from build123d import *

# Parameters (mm, degrees)
F0_W        = 292.1
F0_H        = 474.98
F1_DEPTH    = 12.7
F2_W        = 157.1649909019
F2_H        = 403.2308459282
F3_DEPTH    = 6.35
F4_T1_DEPTH = 445.8279408996
F4_T3_DEPTH = 199.7620858733


# Not quite as in the source:
# - a fillet or chamfer that OpenCascade refuses, or shapes differently, is made with other operations: its cross-section is extruded or revolved along the edge and cut away or added


with BuildPart() as f1:
    # F0 (on Front) → F1 (new body)
    with BuildSketch(Plane.XZ):
        Rectangle(F0_W, F0_H)
    extrude(amount=F1_DEPTH)

    # F2 (on face) → F3 (cut)
    with BuildSketch(Plane.XZ.offset(12.7)):
        Rectangle(F2_W, F2_H)
    extrude(amount=-F3_DEPTH, mode=Mode.SUBTRACT)

    # F4: fillet of radius 8.89 on 4 edges, made by hand

    # F4_s2 → F4_t1 (join)
    with BuildSketch(Plane.XY.offset(-222.9139704498)):
        with BuildLine():
            ThreePointArc((78.582495451, -12.7), (75.3758676252, -8.1121426782), (70.0630764567, -6.35))
            Line((70.0630764567, -6.35), (78.582495451, -6.35))
            Line((78.582495451, -6.35), (78.582495451, -12.7))
        make_face()
        with BuildLine():
            ThreePointArc((-78.582495451, -12.7), (-75.3758676252, -8.1121426782), (-70.0630764567, -6.35))
            Line((-70.0630764567, -6.35), (-78.582495451, -6.35))
            Line((-78.582495451, -6.35), (-78.582495451, -12.7))
        make_face()
    extrude(amount=F4_T1_DEPTH)

    # F4_s4 → F4_t3 (join)
    with BuildSketch(Plane.YZ.offset(-99.8810429367)):
        with BuildLine():
            ThreePointArc((-12.7, 201.6154229641), (-8.1121426782, 198.4087951383), (-6.35, 193.0960039698))
            Line((-6.35, 193.0960039698), (-6.35, 201.6154229641))
            Line((-6.35, 201.6154229641), (-12.7, 201.6154229641))
        make_face()
        with BuildLine():
            ThreePointArc((-12.7, -201.6154229641), (-8.1121426782, -198.4087951383), (-6.35, -193.0960039698))
            Line((-6.35, -193.0960039698), (-6.35, -201.6154229641))
            Line((-6.35, -201.6154229641), (-12.7, -201.6154229641))
        make_face()
    extrude(amount=F4_T3_DEPTH)


solid = f1.part
Model file for the job. Use its own axes, mm. A direction names the side the tool comes from. Coordinates: 2 decimals unless noted, no trailing zeros. Write each loop counter-clockwise with the first axis right and the second up, starting at its lowest first coordinate (ties: lowest second). Pieces come first, ordered by that corner, then holes. Notation, with made-up numbers: (78.5, 40.25) -> (113.5, 40.25) arc R26 cw to (113.5, 68.25) -> close; hole circle Ø4 at (-11, 38.25). An arc over 180 degrees is marked (long way). One line per item, written item: value. Start each with the question number.
1) Which spindle directions (+Z, -Z, +X, -X, +Y, -Y) get a long thin tool onto all of the face, cutting with end or side? Do faces 1 (the face through (-2, 0, 3)), 2 (the face through (-1.1, -8.16, 198.47)). Say none if no direction does.
2) Slice it at B-B on z = -110.5. Write the cut outline in (x, y), then the cut area to 3 significant figures.
3) Probe probe 1 along Y at (x, z) = (-39, 30); probe 2 along X at (y, z) = (-7.25, 107); probe 3 along X at (y, z) = (-8, 124). List the from-to ranges inside material, lowest first.
4) Flat gauge pins, fed straight in: pin 1 Ø6 at (x, z) = (28.5, 188) entering from -Y; pin 2 Ø1.5 at (x, z) = (-76, 89.5) entering from -Y. Where does each tip first touch, or does it go through?
5) Slice it at C-C on y = -9. Write the cut outline in (x, z), then the cut area to 3 significant figures.
6) Slice it at A-A on x = -53.5. Write the cut outline in (y, z), then the cut area to 3 significant figures.
7) Pull direction Z, two halves, no side cores. Call faces 3 (the face through (-1, -6.35, 3)), 4 (the face through (75.44, -8.16, -2.82)), 5 (the face through (146.05, -6, -3)), 6 (the face through (-2, -6, -237.49)): +Z half, -Z half, draft (parallel to the pull), parting line (faces both ways), or undercut.
Answers follow:
1. face 1: +Z, -Z, +X, -X, +Y
1. face 2: -Y
2. outline: (-146.05, -12.7) -> (-78.58, -12.7) arc R8.89 cw to (-70.06, -6.35) -> (70.06, -6.35) arc R8.89 cw to (78.58, -12.7) -> (146.05, -12.7) -> (146.05, 0) -> (-146.05, 0) -> close
2. area: 2,740 mm2
3. probe 1: -6.35 to 0
3. probe 2: -146.05 to -73.96, 73.96 to 146.05
3. probe 3: -146.05 to -75.22, 75.22 to 146.05
4. pin 1: y = -6.35
4. pin 2: y = -9.38
5. outline: (-146.05, -237.49) -> (146.05, -237.49) -> (146.05, 237.49) -> (-146.05, 237.49) -> close; hole (-76.4, -199.43) -> (76.4, -199.43) -> (76.4, 199.43) -> (-76.4, 199.43) -> close
5. area: 77,800 mm2
6. outline: (-12.7, -237.49) -> (0, -237.49) -> (0, 237.49) -> (-12.7, 237.49) -> (-12.7, 201.62) arc R8.89 cw to (-6.35, 193.1) -> (-6.35, -193.1) arc R8.89 cw to (-12.7, -201.62) -> close
6. area: 3,500 mm2
7. face 3: undercut
7. face 4: undercut
7. face 5: draft
7. face 6: -Z half
